Geometry: see drawing. Coordinates: mm, zero at the bounding-box minimum. A direction names the side the tool comes from. Coordinates: 2 decimals unless noted, no trailing zeros. Order: outer loops, then holes, each group sorted by start corner. A loop starts at its lowest first (then second) coordinate and runs counter-clockwise, first axis right, second up.
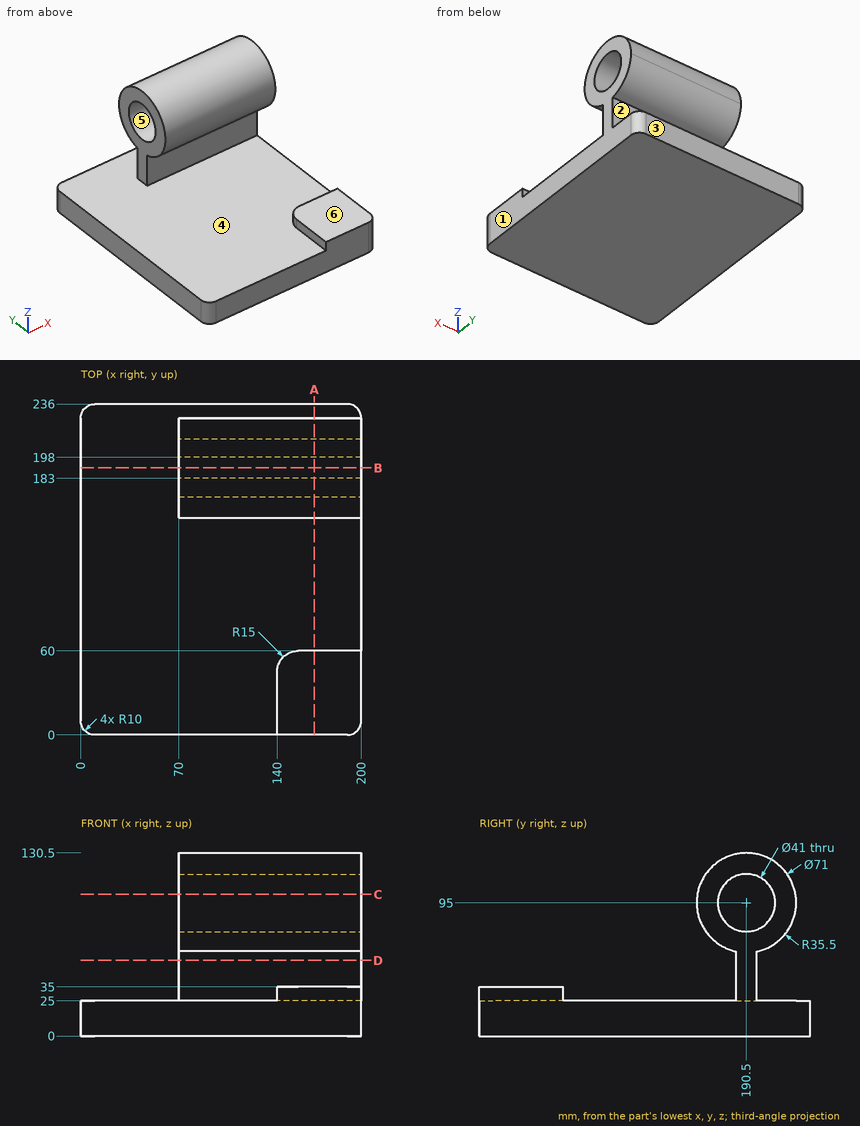
Q1. Set-up query: the marked faces 1 and 2. Return all of +Z, -Z, +X, -X, +Y, -Y with unobstructed straight access to the full face (end or side cutting, diameter ignored); none if empty.
Solutions:
face 1: +Z, -Z, +X, +Y, -Y
face 2: +X, -X, +Y
Q2. Pull-direction query (Y, two-part tool) for the marked faces 3, 4, 5 and 6; classes: pulls with the +Y half, pulls with the -Y half, needs draft (parallel to the pull), parting line crosses it, or undercut.
Solutions:
face 3: pulls with the +Y half
face 4: undercut
face 5: undercut
face 6: needs draft
Q3. Section query A-A on x = 166.5. Output: boundary loops of the cut face in (y, z), plus the area to 3 significant figures.
Solutions:
outline: (0, 0) - (236, 0) - (236, 25) - (198, 25) - (198, 60.3) arc R35.5 ccw to (226, 95) arc R35.5 ccw (long way) to (183, 60.3) - (183, 25) - (60, 25) - (60, 35) - (0, 35) - close; hole circle Ø41 at (190.5, 95)
area: 9,660 mm2
Q4. Material intervals for line 1 along Z through (x, y) = (128, 190); line 2 along Z through (x, y) = (35.5, 66); line 3 along Y through (x, z) = (190.5, 45.5), sorted ascending.
Solutions:
line 1: z = 0 to 74.51, 115.49 to 130.5
line 2: z = 0 to 25
line 3: y = 183 to 198
Q5. Section query C-C on z = 101. Output: boundary loops of the cut face in (x, y).
Solutions:
outline: (70, 155.51) - (200, 155.51) - (200, 170.9) - (70, 170.9) - close; (70, 210.1) - (200, 210.1) - (200, 225.49) - (70, 225.49) - close
Q6. Section query B-B on y = 190.5. Output: boundary loops of the cut face in (x, z).
Solutions:
outline: (0, 0) - (200, 0) - (200, 74.5) - (70, 74.5) - (70, 25) - (0, 25) - close; (70, 115.5) - (200, 115.5) - (200, 130.5) - (70, 130.5) - close
Q7. Pin query (flat end, axial travel): P1, Ø2, axis at x = 146, y = 135, coming from the +Z side; P2, Ø8, axis at y = 33, z = 30, coming from the -X side; P3, Ø1, axis at x = 115, z = 54.5, coming from the +Y side. Return the tip coordinate at first contact, or that it passes through.
Solutions:
P1: stops at z = 25
P2: stops at x = 140
P3: stops at y = 198
Q8. Section query D-D on z = 54. Output: boundary loops of the cut face in (x, y), plus the area to 3 significant figures.
Solutions:
outline: (70, 183) - (200, 183) - (200, 198) - (70, 198) - close
area: 1,950 mm2
